from build123d import *

# Parameters (mm, degrees)
CYLINDER072_R              = 6
CYLINDER072_DEPTH          = 30
CYLINDER071_R              = 2.1
CYLINDER071_DEPTH          = 10
CYLINDER074_R              = 1.6
CYLINDER074_DEPTH          = 15
CYLINDER075_R              = 4
CYLINDER075_DEPTH          = 4
BOX025_W                   = 13
BOX025_H                   = 8
BOX025_DEPTH               = 4
EXTRUDE005_DEPTH           = 3
EXTRUDE005_PLACEMENT_ANGLE = 180
EXTRUDE018_DEPTH           = 10
BOX023_W                   = 51
BOX023_H                   = 26
BOX023_DEPTH               = 4
EXTRUDE017_DEPTH           = 26
CYLINDER073_R              = 4.1
CYLINDER073_DEPTH          = 240
BOX024_W                   = 12
BOX024_H                   = 35
BOX024_DEPTH               = 1
BOX022_W                   = 21
BOX022_H                   = 26
BOX022_DEPTH               = 33


with BuildPart() as cylinder072:
    # Cylinder072 → Cylinder072 (new body)
    with BuildSketch(Plane.XY.offset(10)):
        Circle(CYLINDER072_R)
    extrude(amount=CYLINDER072_DEPTH)


with BuildPart() as fusion032:
    # Cylinder071 → Cylinder071 (new body)
    with BuildSketch(Plane.XY):
        Circle(CYLINDER071_R)
    extrude(amount=CYLINDER071_DEPTH)

    # Fusion032: union Cylinder072
    add(cylinder072.part)


with BuildPart() as fusion032_1:
    # Fusion032 placement: moved
    add(fusion032.part.moved(Location((-14, 12, -29))))


with BuildPart() as cylinder074:
    # Cylinder074 → Cylinder074 (new body)
    with BuildSketch(Plane.XY):
        Circle(CYLINDER074_R)
    extrude(amount=CYLINDER074_DEPTH)


with BuildPart() as fusion009:
    # Cone → Cone (revolve)
    with BuildSketch(Plane(origin=(0, 0, 15), x_dir=(1, 0, 0), z_dir=(0, -1, 0))):
        Polygon((0, 0), (1.6, 0), (2.5, 2.5), (0, 2.5), align=None)
    revolve(axis=Axis((0, 0, 15), (0, 0, 1)))

    # Fusion009: union Cylinder074
    add(cylinder074.part)


with BuildPart() as fusion009_1:
    # Fusion009 placement: moved
    add(fusion009.part.moved(Location((9, 11, -7))))


with BuildPart() as cylinder075:
    # Cylinder075 → Cylinder075 (new body)
    with BuildSketch(Plane(origin=(9, 11, -8), x_dir=(1, 0, 0), z_dir=(0, 0, 1))):
        Circle(CYLINDER075_R)
    extrude(amount=CYLINDER075_DEPTH)


with BuildPart() as fusion010:
    # Box025 → Box025 (new body)
    with BuildSketch(Plane(origin=(9, 7, -8), x_dir=(1, 0, 0), z_dir=(0, 0, 1))):
        with Locations((6.5, 4)):
            Rectangle(BOX025_W, BOX025_H)
    extrude(amount=BOX025_DEPTH)

    # Fusion010: union Cylinder075
    add(cylinder075.part)


with BuildPart() as extrude005:
    # Sketch004 → Extrude005 (new body)
    with BuildSketch(Plane.XZ):
        Polygon((-22, -19), (-7, -19), (-7, -4), align=None)
    extrude(amount=-EXTRUDE005_DEPTH)


with BuildPart() as extrude005_1:
    # Extrude005 placement: moved
    add(extrude005.part.moved(Location((7, 0, 0))).rotate(Axis((7, 0, 0), (0, 0, 1)), EXTRUDE005_PLACEMENT_ANGLE))


with BuildPart() as extrude018:
    # Sketch003 → Extrude018 (new body)
    with BuildSketch(Plane.XY):
        with BuildLine():
            ThreePointArc((35.736492, 10), (36.2, 15), (35.736492, 20))
            ThreePointArc((35.736492, 20), (33.490746, 22.111711), (31.244999, 20))
            ThreePointArc((31.244999, 10), (31.8, 15), (31.244999, 20))
            ThreePointArc((31.244999, 10), (33.490746, 7.888289), (35.736492, 10))
        make_face()
    extrude(amount=-EXTRUDE018_DEPTH)


with BuildPart() as extrude018_1:
    # Extrude018 placement: moved
    add(extrude018.part.moved(Location((-12, -3, -17))))


with BuildPart() as cut017:
    # Box023 → Box023 (new body)
    with BuildSketch(Plane(origin=(-22, 0, -23), x_dir=(1, 0, 0), z_dir=(0, 0, 1))):
        with Locations((25.5, 13)):
            Rectangle(BOX023_W, BOX023_H)
    extrude(amount=BOX023_DEPTH)

    # Cut017: cut Extrude018
    add(extrude018_1.part, mode=Mode.SUBTRACT)


with BuildPart() as cut017_1:
    # Cut017 placement: moved
    add(cut017.part.moved(Location((0, -3, 0))))


with BuildPart() as extrude017:
    # Sketch016 → Extrude017 (new body)
    with BuildSketch(Plane.XZ):
        Polygon((-22, -19), (-7, -19), (-7, 10), align=None)
    extrude(amount=-EXTRUDE017_DEPTH)


with BuildPart() as extrude017_1:
    # Extrude017 placement: moved
    add(extrude017.part.moved(Location((0, -3, 0))))


with BuildPart() as cylinder073:
    # Cylinder073 → Cylinder073 (new body)
    with BuildSketch(Plane(origin=(0, -7, 0), x_dir=(1, 0, 0), z_dir=(0, 1, 0))):
        Circle(CYLINDER073_R)
    extrude(amount=CYLINDER073_DEPTH)


with BuildPart() as box024:
    # Box024 → Box024 (new body)
    with BuildSketch(Plane(origin=(3, -6, 0), x_dir=(1, 0, 0), z_dir=(0, 0, 1))):
        with Locations((6, 17.5)):
            Rectangle(BOX024_W, BOX024_H)
    extrude(amount=BOX024_DEPTH)


with BuildPart() as cut022:
    # Box022 → Box022 (new body)
    with BuildSketch(Plane(origin=(-7, -3, -23), x_dir=(1, 0, 0), z_dir=(0, 0, 1))):
        with Locations((10.5, 13)):
            Rectangle(BOX022_W, BOX022_H)
    extrude(amount=BOX022_DEPTH)

    # Cut018: cut Box024
    add(box024.part, mode=Mode.SUBTRACT)

    # Cut019: cut Cylinder073
    add(cylinder073.part, mode=Mode.SUBTRACT)

    # Fusion031: union Cut017, Extrude017
    add(cut017_1.part)
    add(extrude017_1.part)

    # Fusion011: union Extrude005
    add(extrude005_1.part)

    # Cut020: cut Fusion010
    add(fusion010.part, mode=Mode.SUBTRACT)

    # Cut021: cut Fusion009
    add(fusion009_1.part, mode=Mode.SUBTRACT)

    # Cut022: cut Fusion032
    add(fusion032_1.part, mode=Mode.SUBTRACT)


with BuildPart() as cut022_1:
    # Cut022 placement: moved
    add(cut022.part.moved(Location((0, -9, 0))))


solid = cut022_1.part
For this review, take the finished solid that the model builds, in its own axes (mm). A direction names the side the tool comes from. Round coordinates to 2 decimals unless told otherwise and drop trailing zeros. Loops run counter-clockwise (first coordinate to the right, second up) from the corner with the lowest first, then second, coordinate; pieces in that order, holes last. Notation, with made-up numbers: (3, -24) - (15, -24) arc R36 cw to (15, 13) - close; hole circle Ø2 at (8, 64). An arc over 180 degrees is marked (long way). Answer as CSV lines item,"result".
(1) Wall thickness on line 1 (Z direction, x = 13.5, y = 7.75); line 2 (Y direction, x = -14, z = -13); line 3 (Z direction, x = 0, y = -3.75): over which ranges is each line inside the solid? List them lowest first.
Checked values:
line 1,"z = -23 to 0, 1 to 10"
line 2,"y = -12 to -3, 9 to 14"
line 3,"z = -23 to -4.1, 4.1 to 10"
(2) Tool access review of faces 5 (the face through (14, 1, 5)), 6 (the face through (11, 1, 0)), 7 (the face through (7.4, 2.07, 4.45)): name each direction out of +Z, -Z, +X, -X, +Y, -Y from which nothing blocks a thin tool from reaching the whole face with its end or side.
Checked values:
face 5,"+Z, +X, +Y, -Y"
face 6,"+X, +Y, -Y"
face 7,"+Z"
(3) Consider section A-A on x = 13. Give the boundary of the cut face in (y, z), then the cut area to 3 significant figures.
Checked values:
outline,"(-12, -23) - (14, -23) - (14, 0) - (-12, 0) - close; (-12, 1) - (14, 1) - (14, 10) - (-12, 10) - close; hole (-2, -8) - (6, -8) - (6, -4) - (-2, -4) - close"
area,"800 mm2"
(4) Consider section D-D on z = -11. Give the boundary of the cut face in (x, y), then the cut area to 3 significant figures.
Checked values:
outline,"(-17.86, -12) - (21, -12) - (21, -9) - (14, -9) - (14, 14) - (-17.86, 14) - (-17.86, 7.59) arc R6 cw (long way) to (-17.86, -1.59) - close"
area,"750 mm2"
(5) Consider section B-B on z = -20. Give the number of separate pieces and of enclosed holes in the cut face, then the cut area to 3 significant figures.
Checked values:
separate pieces,"1"
enclosed holes,"2"
area,"1,250 mm2"
(6) Mouldability with a two-part tool opening along Y and no side actions: class faces 1 (the face through (4, -12, -10)), 2 (the face through (11, -2, -6)), 3 (the face through (19.8, -0.1, -21)), 4 (the face through (-22, 1, -21)) as +Y half, -Y half, draft (parallel to the pull), parting line (faces both ways), or undercut.
Checked values:
face 1,"-Y half"
face 2,"undercut"
face 3,"undercut"
face 4,"draft"
(7) Consider section C-C on x = 0. Give the boundary of the cut face in (y, z), then the cut area to 3 significant figures.
Checked values:
outline,"(-12, -23) - (14, -23) - (14, -4.1) - (-12, -4.1) - close; (-12, 4.1) - (14, 4.1) - (14, 10) - (-12, 10) - close"
area,"645 mm2"
(8) Insertion check: P1, Ø11, axis at x = -14, y = 3, coming from the +Z side; P2, Ø5, axis at y = 3.5, z = -14, coming from the +X side; P3, Ø2, axis at y = 10.5, z = -9, coming from the -X side. Each pin has a flat end and moves straight along its axis. Give the tip position at first contact, or say it passes through.
Checked values:
P1,"stops at z = -19"
P2,"stops at x = 14"
P3,"stops at x = -17.34"
